from build123d import *

# Parameters (mm, degrees)
BOSS_EXTRUDE1_DEPTH = 2
SKETCH2_R           = 1.6
CUT_EXTRUDE1_DEPTH  = 2
SKETCH5_R           = 2.5
CUT_EXTRUDE2_DEPTH  = 1
SKETCH6_W           = 25
SKETCH6_H           = 3.6
SKETCH6_W_2         = 23
SKETCH6_H_2         = 1.6
BOSS_EXTRUDE2_DEPTH = 4
SKETCH7_W           = 18.6
SKETCH7_H           = 4
CUT_EXTRUDE3_DEPTH  = 15
SKETCH9_W           = 3.6
SKETCH9_H           = 30
SKETCH9_W_2         = 1.6
SKETCH9_H_2         = 28
BOSS_EXTRUDE4_DEPTH = 4
SKETCH10_W          = 4
SKETCH10_H          = 25.6
CUT_EXTRUDE4_DEPTH  = 4
SKETCH11_W          = 22.4
SKETCH11_H          = 27.5
SKETCH11_W_2        = 20.4
SKETCH11_H_2        = 25.5
BOSS_EXTRUDE5_DEPTH = 4
SKETCH12_W          = 20.4
SKETCH12_H          = 25.5
BOSS_EXTRUDE6_DEPTH = 3
SKETCH13_W          = 18.4
SKETCH13_H          = 23.5
CUT_EXTRUDE5_DEPTH  = 3
SKETCH14_W          = 4
SKETCH14_H          = 22.5
CUT_EXTRUDE6_DEPTH  = 30
SKETCH15_W          = 17.4
SKETCH15_H          = 4
CUT_EXTRUDE7_DEPTH  = 30
SKETCH16_W          = 22.3
SKETCH16_H          = 78.2
SKETCH16_W_2        = 20.3
SKETCH16_H_2        = 76.2
BOSS_EXTRUDE7_DEPTH = 10
SKETCH17_W          = 17.3
SKETCH17_H          = 10
CUT_EXTRUDE8_DEPTH  = 10
CUT_EXTRUDE9_REACH  = 95.2
SKETCH18_W          = 17.3
SKETCH18_H          = 10
CUT_EXTRUDE10_REACH = 96.44
SKETCH19_W          = 10
SKETCH19_H          = 73.2
CUT_EXTRUDE11_REACH = 90.088
SKETCH20_W          = 10
SKETCH20_H          = 73.2
SKETCH21_W          = 1.5
SKETCH21_H          = 1.5
BOSS_EXTRUDE8_DEPTH = 8


with BuildPart() as part:
    # 3DSketch1 → Boss-Extrude1 (new body)
    with BuildSketch(Plane(origin=(-20, 20.801620861, 0), x_dir=(0.3746178943835793, -0.927179288599359, 0), z_dir=(0, 0, 1))):
        Polygon((0, 0), (14.984715775, 37.087171544), (27.501636171, 32.02982997), (32.93359564, 45.473929654), (99.690504419, 18.501441259), (94.258544951, 5.057341574), (106.775465347, 0), (91.790749571, -37.087171544), (79.273829175, -32.02982997), (73.841869707, -45.473929654), (7.084960928, -18.501441259), (12.516920396, -5.057341574), align=None)
    extrude(amount=-BOSS_EXTRUDE1_DEPTH)

    # Sketch2 → Cut-Extrude1 (cut)
    with BuildSketch(Plane.XY):
        with Locations((-20, 1.301620861)):
            Circle(SKETCH2_R)
        with Locations((20, 1.301620861)):
            Circle(SKETCH2_R)
        with Locations((20, -58.698379139)):
            Circle(SKETCH2_R)
        with Locations((-20, -58.698379139)):
            Circle(SKETCH2_R)
    extrude(amount=-CUT_EXTRUDE1_DEPTH, mode=Mode.SUBTRACT)

    # Sketch5 → Cut-Extrude2 (cut)
    with BuildSketch(Plane.XY):
        with Locations((-20, 1.301620861)):
            Circle(SKETCH5_R)
        with Locations((20, 1.301620861)):
            Circle(SKETCH5_R)
        with Locations((20, -58.698379139)):
            Circle(SKETCH5_R)
        with Locations((-20, -58.698379139)):
            Circle(SKETCH5_R)
    extrude(amount=-CUT_EXTRUDE2_DEPTH, mode=Mode.SUBTRACT)

    # Sketch6 → Boss-Extrude2 (add)
    with BuildSketch(Plane.XY):
        with Locations((0, 12.001620861)):
            Rectangle(SKETCH6_W, SKETCH6_H)
        with Locations((0, 12.001620861)):
            Rectangle(SKETCH6_W_2, SKETCH6_H_2, mode=Mode.SUBTRACT)
    extrude(amount=BOSS_EXTRUDE2_DEPTH)

    # Sketch7 → Cut-Extrude3 (cut)
    with BuildSketch(Plane(origin=(0, 13.801620861, 0), x_dir=(1, 0, 0), z_dir=(0, 1, 0))):
        with Locations((0, -2)):
            Rectangle(SKETCH7_W, SKETCH7_H)
    extrude(amount=-CUT_EXTRUDE3_DEPTH, mode=Mode.SUBTRACT)

    # Sketch9 → Boss-Extrude4 (add)
    with BuildSketch(Plane.XY):
        with Locations((28.7, -13.698379139)):
            Rectangle(SKETCH9_W, SKETCH9_H)
        with Locations((28.7, -13.698379139)):
            Rectangle(SKETCH9_W_2, SKETCH9_H_2, mode=Mode.SUBTRACT)
    extrude(amount=BOSS_EXTRUDE4_DEPTH)

    # Sketch10 → Cut-Extrude4 (cut)
    with BuildSketch(Plane(origin=(30.5, 0, 0), x_dir=(0, 0, -1), z_dir=(1, 0, 0))):
        with Locations((-2, -13.698379139)):
            Rectangle(SKETCH10_W, SKETCH10_H)
    extrude(amount=-CUT_EXTRUDE4_DEPTH, mode=Mode.SUBTRACT)

    # Sketch11 → Boss-Extrude5 (add)
    with BuildSketch(Plane.XY):
        with Locations((6.3, -29.448379139)):
            Rectangle(SKETCH11_W, SKETCH11_H)
        with Locations((6.3, -29.448379139)):
            Rectangle(SKETCH11_W_2, SKETCH11_H_2, mode=Mode.SUBTRACT)
    extrude(amount=BOSS_EXTRUDE5_DEPTH)

    # Sketch12 → Boss-Extrude6 (add)
    with BuildSketch(Plane.XY):
        with Locations((6.3, -29.448379139)):
            Rectangle(SKETCH12_W, SKETCH12_H)
    extrude(amount=BOSS_EXTRUDE6_DEPTH)

    # Sketch13 → Cut-Extrude5 (cut)
    with BuildSketch(Plane.XY.offset(3)):
        with Locations((6.3, -29.448379139)):
            Rectangle(SKETCH13_W, SKETCH13_H)
    extrude(amount=-CUT_EXTRUDE5_DEPTH, mode=Mode.SUBTRACT)

    # Sketch14 → Cut-Extrude6 (cut)
    with BuildSketch(Plane.ZY.offset(4.9)):
        with Locations((2, -29.448379139)):
            Rectangle(SKETCH14_W, SKETCH14_H)
    extrude(amount=-CUT_EXTRUDE6_DEPTH, mode=Mode.SUBTRACT)

    # Sketch15 → Cut-Extrude7 (cut)
    with BuildSketch(Plane.XZ.offset(43.198379139)):
        with Locations((6.3, 2)):
            Rectangle(SKETCH15_W, SKETCH15_H)
    extrude(amount=-CUT_EXTRUDE7_DEPTH, mode=Mode.SUBTRACT)

    # Sketch16 → Boss-Extrude7 (add)
    with BuildSketch(Plane.XY):
        with Locations((-6.35, -31.298379139)):
            Rectangle(SKETCH16_W, SKETCH16_H)
        with Locations((-6.35, -31.298379139)):
            Rectangle(SKETCH16_W_2, SKETCH16_H_2, mode=Mode.SUBTRACT)
    extrude(amount=BOSS_EXTRUDE7_DEPTH)

    # Sketch17 → Cut-Extrude8 (cut)
    with BuildSketch(Plane.XZ.offset(70.398379139)):
        with Locations((-6.35, 5)):
            Rectangle(SKETCH17_W, SKETCH17_H)
    extrude(amount=-CUT_EXTRUDE8_DEPTH, mode=Mode.SUBTRACT)

    # Sketch18 → Cut-Extrude9 (cut, up to next)
    with BuildSketch(Plane(origin=(0, 7.801620861, 0), x_dir=(1, 0, 0), z_dir=(0, 1, 0)), mode=Mode.PRIVATE) as cut_extrude9_sk1:
        with Locations((-6.35, -5)):
            Rectangle(SKETCH18_W, SKETCH18_H)
    cut_extrude9_tool1 = extrude(cut_extrude9_sk1.sketch, amount=-CUT_EXTRUDE9_REACH, mode=Mode.PRIVATE) & part.part
    add(cut_extrude9_tool1.solids().sort_by_distance((-6.35, 7.801621, 5))[0], mode=Mode.SUBTRACT)

    # Sketch19 → Cut-Extrude10 (cut, up to next)
    with BuildSketch(Plane.ZY.offset(17.5), mode=Mode.PRIVATE) as cut_extrude10_sk1:
        with Locations((5, -31.298379139)):
            Rectangle(SKETCH19_W, SKETCH19_H)
    cut_extrude10_tool1 = extrude(cut_extrude10_sk1.sketch, amount=-CUT_EXTRUDE10_REACH, mode=Mode.PRIVATE) & part.part
    add(cut_extrude10_tool1.solids().sort_by_distance((-17.5, -31.298379, 5))[0], mode=Mode.SUBTRACT)

    # Sketch20 → Cut-Extrude11 (cut, up to next)
    with BuildSketch(Plane(origin=(4.8, 0, 0), x_dir=(0, 0, -1), z_dir=(1, 0, 0)), mode=Mode.PRIVATE) as cut_extrude11_sk1:
        with Locations((-5, -31.298379139)):
            Rectangle(SKETCH20_W, SKETCH20_H)
    cut_extrude11_tool1 = extrude(cut_extrude11_sk1.sketch, amount=-CUT_EXTRUDE11_REACH, mode=Mode.PRIVATE) & part.part
    add(cut_extrude11_tool1.solids().sort_by_distance((4.8, -31.298379, 5))[0], mode=Mode.SUBTRACT)

    # Sketch21 → Boss-Extrude8 (add)
    with BuildSketch(Plane.XY):
        with Locations((-15.75, 6.051620861)):
            Rectangle(SKETCH21_W, SKETCH21_H)
        with Locations((3.05, 6.051620861)):
            Rectangle(SKETCH21_W, SKETCH21_H)
        with Locations((3.05, -68.648379139)):
            Rectangle(SKETCH21_W, SKETCH21_H)
        with Locations((-15.75, -68.648379139)):
            Rectangle(SKETCH21_W, SKETCH21_H)
    extrude(amount=BOSS_EXTRUDE8_DEPTH)


solid = part.part
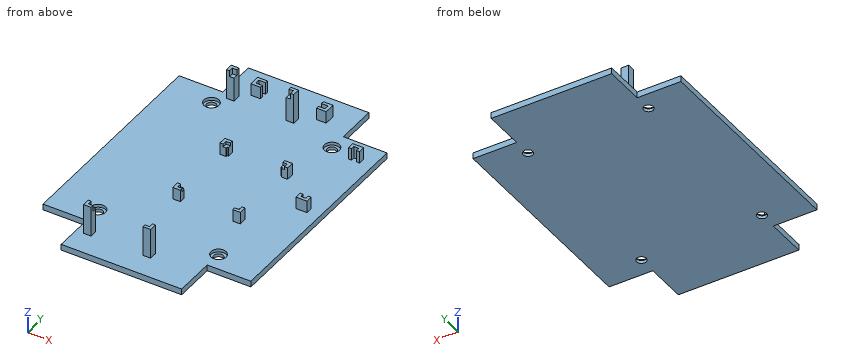
Can you work these out from the model? Positions are in its coordinate system, mm. Coordinates: 2 decimals unless noted, no trailing zeros. Order: outer loops, then holes, each group sorted by start corner. A loop starts at its lowest first (then second) coordinate and runs counter-clockwise, first axis right, second up. Notation, with made-up numbers: M -22,-19.75 L -13,-19.75 A18 cw -13,-9.75 Z; hole C 4,-0.5 d3. An arc over 180 degrees is marked long. Answer as CSV lines item,"result".
(1) Suppose I cut it at C-C on y = -37. Please give me the cut outline in (x, z).
Geometry check:
outline,"M -34.5,-2 L 34.5,-2 L 34.5,0 L -34.5,0 Z"
(2) Suppose I cut it at B-B on z = 1.75. Count the separate pieces of the cut face and the enclosed holes in it, plus the area to 3 significant figures.
Geometry check:
separate pieces,"12"
enclosed holes,"0"
area,"77.0 mm^2"
(3) Suppose I cut it at D-D on x = 25. Please give me the cut outline in (y, z).
Geometry check:
outline,"M -64.7,-2 L 7.3,-2 L 7.3,0 L -64.7,0 Z"
(4) I'm going to push flat-ended pins straight in: pin 1 (0.6 mm diameter, centred on x = -4, z = 2.5, fed in from -Y); pin 2 (0.8 mm diameter, centred on y = -17.5, z = 2.5, fed in from -X); pin 3 (0.8 mm diameter, centred on y = -69, z = 9.5, fed in from +X); pin 4 (12 mm diameter, centred on x = -13.5, y = -66.5, fed in from +Z). Where does each tip first touch, or does it pass through?
Geometry check:
pin 1,"y = -43.2"
pin 2,"x = -4.9"
pin 3,"x = 4.8"
pin 4,"z = 10"
(5) Please list where these lines run through material, in increasing order: L1, parallel to Y at x = 4, z = 6.25; L2, parallel to X at y = -65.5, z = -1; L3, parallel to X at y = -27.5, z = 0.75.
Geometry check:
L1,"-70.4 to -67.9, 5.3 to 7.8"
L2,"-20 to 20"
L3,"26.9 to 27.9, 29.5 to 30.5"
(6) Suppose I cut it at A-A on z = 6.25. Please give me the cut outline in (x, y).
Geometry check:
outline,"M -17.5,-70.4 L -15,-70.4 L -15,-67.9 L -17.5,-67.9 Z; M -17.5,5.3 L -15,5.3 L -15,7.8 L -17.5,7.8 Z; M 2.3,-70.4 L 4.8,-70.4 L 4.8,-67.9 L 2.3,-67.9 Z; M 2.3,5.3 L 4.8,5.3 L 4.8,7.8 L 2.3,7.8 Z"
